The model under review builds one solid part; all positions refer to its coordinate system, in mm. A direction names the side the tool comes from. Round coordinates to 2 decimals unless told otherwise and drop trailing zeros. Order: outer loops, then holes, each group sorted by start corner. A loop starts at its lowest first (then second) coordinate and runs counter-clockwise, first axis right, second up.
```python
from build123d import *

# Parameters (mm, degrees)
BOSS_EXTRUDE1_DEPTH = 76.2
SKETCH3_R           = 3.175
BOSS_EXTRUDE3_DEPTH = 10.16
FILLET2_R           = 3.175
FILLET3_R           = 8.255


# Some blends are built 0.0001 mm under size
with BuildPart() as part:
    # Sketch1 → Boss-Extrude1 (new body)
    with BuildSketch(Plane(origin=(0, 0, 0), x_dir=(1, 0, 0), z_dir=(0, 1, 0))):
        Polygon((44.45, 38.1), (76.2, 38.1), (76.2, 0), (82.55, 0), (82.55, 38.1), (82.55, 50.8), (0, 50.8), (0, 38.1), (0, 0), (6.35, 0), (6.35, 38.1), (38.1, 38.1), (38.1, 0), (44.45, 0), align=None)
    extrude(amount=BOSS_EXTRUDE1_DEPTH)

    # Sketch3 → Boss-Extrude3 (add)
    with BuildSketch(Plane.XY):
        with Locations((3.175, 73.025)):
            Circle(SKETCH3_R)
        with Locations((3.175, 3.175)):
            Circle(SKETCH3_R)
        with Locations((41.275, 3.175)):
            Circle(SKETCH3_R)
        with Locations((79.375, 3.175)):
            Circle(SKETCH3_R)
        with Locations((41.275, 73.025)):
            Circle(SKETCH3_R)
        with Locations((79.375, 73.025)):
            Circle(SKETCH3_R)
    extrude(amount=BOSS_EXTRUDE3_DEPTH)

    # Fillet2
    fillet2_edges = [part.edges().sort_by_distance(p)[0] for p in [
        (6.35, 0, -19.05),
        (22.225, 0, -38.1),
        (38.1, 0, -19.05),
        (44.45, 0, -19.05),
        (60.325, 0, -38.1),
        (76.2, 0, -19.05),
        (82.55, 0, -25.4),
        (41.275, 0, -50.8),
        (0, 0, -25.4),
        (41.275, 76.2, -50.8),
        (82.55, 76.2, -25.4),
        (76.2, 76.2, -19.05),
        (60.325, 76.2, -38.1),
        (44.45, 76.2, -19.05),
        (38.1, 76.2, -19.05),
        (22.225, 76.2, -38.1),
        (6.35, 76.2, -19.05),
        (0, 76.2, -25.4),
    ]]
    fillet(fillet2_edges, radius=FILLET2_R - 0.0001)  # a hair under: the kernel refuses the full size

    # Fillet3
    # the kernel refuses this fillet: 8.255 mm, written as the material it takes off along each edge
    with BuildSketch(Plane(origin=(74.295, 0, -42.545), x_dir=(0, 0, -1), z_dir=(-1, 0, 0))) as fillet3_piece_1:
        with BuildLine():
            CenterArc((5.0801, -3.1749), 3.1749, 0, 90)
            Line((8.255, -3.1749), (8.255, 0))
            Line((8.255, 0), (5.0801, 0))
        make_face()
    revolve(axis=Axis((74.295, 0, -42.545), (0, -1, 0)), revolution_arc=90, mode=Mode.SUBTRACT)
    with BuildSketch(Plane(origin=(8.255, 0, -42.545), x_dir=(-1, 0, 0), z_dir=(0, 0, 1))) as fillet3_piece_2:
        with BuildLine():
            CenterArc((5.0801, -3.1749), 3.1749, 0, 90)
            Line((8.255, -3.1749), (8.255, 0))
            Line((8.255, 0), (5.0801, 0))
        make_face()
    revolve(axis=Axis((8.255, 0, -42.545), (0, -1, 0)), revolution_arc=90, mode=Mode.SUBTRACT)
    with BuildSketch(Plane(origin=(74.295, 76.2, -42.545), x_dir=(1, 0, 0), z_dir=(0, 0, 1))) as fillet3_piece_3:
        with BuildLine():
            CenterArc((5.0801, -3.1749), 3.1749, 0, 90)
            Line((8.255, -3.1749), (8.255, 0))
            Line((8.255, 0), (5.0801, 0))
        make_face()
    revolve(axis=Axis((74.295, 76.2, -42.545), (0, 1, 0)), revolution_arc=90, mode=Mode.SUBTRACT)
    with BuildSketch(Plane(origin=(8.255, 76.2, -42.545), x_dir=(0, 0, -1), z_dir=(1, 0, 0))) as fillet3_piece_4:
        with BuildLine():
            CenterArc((5.0801, -3.1749), 3.1749, 0, 90)
            Line((8.255, -3.1749), (8.255, 0))
            Line((8.255, 0), (5.0801, 0))
        make_face()
    revolve(axis=Axis((8.255, 76.2, -42.545), (0, 1, 0)), revolution_arc=90, mode=Mode.SUBTRACT)
    with BuildSketch(Plane(origin=(0, 0, -50.8), x_dir=(1, 0, 0), z_dir=(0, 1, 0)), Plane(origin=(82.55, 0, -50.8), x_dir=(0, 0, 1), z_dir=(0, 1, 0))) as fillet3_piece_5:
        with BuildLine():
            CenterArc((FILLET3_R, -FILLET3_R), FILLET3_R, 90, 90)
            Line((0, -FILLET3_R), (0, 0))
            Line((0, 0), (FILLET3_R, 0))
        make_face()
    extrude(amount=76.2, mode=Mode.SUBTRACT)


solid = part.part
```
(1) Consider section B-B (x = 13). Write out the cut boundary in (y, z), and give its area (3 significant figures).
Data:
outline: (0, -47.63) arc R3.17 ccw to (3.17, -50.8) - (73.03, -50.8) arc R3.17 ccw to (76.2, -47.63) - (76.2, -41.27) arc R3.17 ccw to (73.03, -38.1) - (3.17, -38.1) arc R3.17 ccw to (0, -41.27) - close
area: 959 mm2
(2) For faces 3 (the cylindrical face through (39.05, 75.29, -20.35)), 4 (the flat face through (41, 0, -45)), 5 (the cylindrical face through (77.15, 0.91, -20.35)), 6 (the flat face through (38.1, 38, -19)), 7 (the cylindrical face through (2.487, 69.926, 5.009)), list the 3-axis set-ups (+Z, -Z, +X, -X, +Y, -Y) from which the entire face can be reached by the end or side of a thin tool; tool diameter is ignored.
Data:
face 3: +Z, +Y
face 4: +Z, -Z, +X, -X, -Y
face 5: +Z, -Y
face 6: +Z, +Y, -Y
face 7: +Z
(3) Insertion check: pin 1 (3 mm diameter, centred on x = 42, y = 37, fed in from +Z); pin 2 (3 mm diameter, centred on x = 31.5, y = 35, fed in from +Z). Each pin has a flat end and moves straight along its axis. Give the tip position at first contact, or say it passes through.
Data:
pin 1: stops at z = 0
pin 2: stops at z = -38.1
(4) To check wall thickness, follow probe 1 along X at (y, z) = (25, -32); probe 2 along Z at (x, y) = (12.5, 56); probe 3 along Z at (x, y) = (42.5, 63.5). State the ranges of each line that lie inside material, in increasing order.
Data:
probe 1: x = 0 to 6.35, 38.1 to 44.45, 76.2 to 82.55
probe 2: z = -50.8 to -38.1
probe 3: z = -50.8 to 0
(5) Consider section A-A (z = -8.5). State how many separate pieces and enclosed holes the cut face has, and give its area (3 significant figures).
Data:
separate pieces: 3
enclosed holes: 0
area: 1,430 mm2
(6) Consider section C-C (y = 59). Write out the cut boundary in (x, z) (3 decimals).
Data:
outline: (0, -42.545) arc R8.255 ccw to (8.255, -50.8) - (74.295, -50.8) arc R8.255 ccw to (82.55, -42.545) - (82.55, 0) - (76.2, 0) - (76.2, -38.1) - (44.45, -38.1) - (44.45, 0) - (38.1, 0) - (38.1, -38.1) - (6.35, -38.1) - (6.35, 0) - (0, 0) - close
(7) Draft analysis for pull direction X (two halves, no side actions). For faces 1 (the cylindrical face through (39.05, 0.91, -20.35)), 2 (the flat face through (79, 3, 10.16)), state which applies: pulls with the +X half, pulls with the -X half, needs draft (parallel to the pull), parting line crosses it, or undercut.
Data:
face 1: undercut
face 2: needs draft
